from build123d import *

# Parameters (mm, degrees)
CARTRIDGE_BARREL_SKETCH_R         = 16
CARTRIDGE_BARREL_DEPTH            = 17
SIX_MILLIMETRE_FLANGE_SKETCH_R    = 20
SIX_MILLIMETRE_FLANGE_DEPTH       = 6
BEARING_BORE_SKETCH_R             = 14
BEARING_BORE_DEPTH                = 19.6
OUTER_RACE_SHOULDER_EXIT_SKETCH_R = 13
OUTER_RACE_SHOULDER_EXIT_DEPTH    = 3.6
M3_TAPPED_HOLE_PATTERN_SKETCH_R   = 1.5
M3_TAPPED_HOLE_PATTERN_DEPTH      = 6.2


with BuildPart() as part:
    # Cartridge barrel sketch → Cartridge barrel (new body)
    with BuildSketch(Plane(origin=(0, -237.5, 0), x_dir=(1, 0, 0), z_dir=(0, 1, 0))):
        with Locations(Location((-19.009182883, 53.244882879, 0), (0, 0, 270))):
            Circle(CARTRIDGE_BARREL_SKETCH_R)
    extrude(amount=CARTRIDGE_BARREL_DEPTH)

    # Six millimetre flange sketch → Six millimetre flange (add)
    with BuildSketch(Plane(origin=(0, -220.5, 0), x_dir=(1, 0, 0), z_dir=(0, 1, 0))):
        with Locations(Location((-19.009182883, 53.244882879, 0), (0, 0, 270))):
            Circle(SIX_MILLIMETRE_FLANGE_SKETCH_R)
    extrude(amount=SIX_MILLIMETRE_FLANGE_DEPTH)

    # Bearing bore sketch → Bearing bore (cut)
    with BuildSketch(Plane(origin=(0, -237.6, 0), x_dir=(1, 0, 0), z_dir=(0, 1, 0))):
        with Locations(Location((-19.009182883, 53.244882879, 0), (0, 0, 270))):
            Circle(BEARING_BORE_SKETCH_R)
    extrude(amount=BEARING_BORE_DEPTH, mode=Mode.SUBTRACT)

    # Outer race shoulder exit sketch → Outer race shoulder exit (cut)
    with BuildSketch(Plane(origin=(0, -218, 0), x_dir=(1, 0, 0), z_dir=(0, 1, 0))):
        with Locations(Location((-19.009182883, 53.244882879, 0), (0, 0, 270))):
            Circle(OUTER_RACE_SHOULDER_EXIT_SKETCH_R)
    extrude(amount=OUTER_RACE_SHOULDER_EXIT_DEPTH, mode=Mode.SUBTRACT)

    # M3 tapped hole pattern sketch → M3 tapped hole pattern (cut)
    with BuildSketch(Plane(origin=(0, -220.6, 0), x_dir=(1, 0, 0), z_dir=(0, 1, 0))):
        with Locations(Location((-6.493392856, 40.729092852, 0), (0, 0, 270))):
            Circle(M3_TAPPED_HOLE_PATTERN_SKETCH_R)
        with Locations(Location((-31.52497291, 40.729092852, 0), (0, 0, 270))):
            Circle(M3_TAPPED_HOLE_PATTERN_SKETCH_R)
        with Locations(Location((-31.52497291, 65.760672906, 0), (0, 0, 270))):
            Circle(M3_TAPPED_HOLE_PATTERN_SKETCH_R)
        with Locations(Location((-6.493392856, 65.760672906, 0), (0, 0, 270))):
            Circle(M3_TAPPED_HOLE_PATTERN_SKETCH_R)
    extrude(amount=M3_TAPPED_HOLE_PATTERN_DEPTH, mode=Mode.SUBTRACT)


solid = part.part
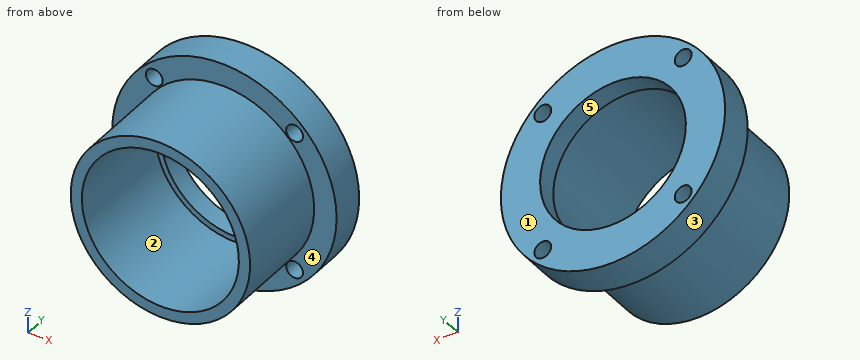
The listing builds one solid part. Answer for the finished solid, in the listing's coordinates (mm). Face numbers are marked on the shaded views. A direction names the side the tool comes from. Round coordinates to 2 decimals unless told otherwise and drop trailing zeros. Write each loop counter-clockwise with the first axis right and the second up, starting at its lowest first coordinate (ties: lowest second). Pieces come first, ordered by that corner, then holes. Notation, with made-up numbers: (15, -30) - (36, -30) arc R18 cw to (36, -20) - close; hole circle Ø10 at (6.5, -8). An arc over 180 degrees is marked (long way). Use a Markdown table: item, result. Add a question column.
1. The part is cut by section A-A (z = -53.5). Write down the section's boundary in (x, y), and give its area (3 significant figures).
2. Flat-ended cylindrical pins translate along their axes: P1, Ø4, axis at y = -227, z = -62.5, coming from the -X side; P2, Ø10, axis at x = -22.5, y = -231, coming from the +Z side; P3, Ø1, axis at x = -16, y = -233.5, coming from the -Z side. Find the tip coordinate at first contact, or state that the pin passes through.
3. The part is cut by section D-D (y = -219.25). Write down the section's boundary in (x, z), and give its area (3 significant figures).
4. The part is cut by section C-C (z = -41). Write down the section's boundary in (x, y).
5. For a pull along X with two mould halves and no side action, classify the marked faces 3, 4 and 5 as +X half, -X half, draft (parallel to the pull), parting line (faces both ways), or undercut.
6. Consider line 1 (Z direction, x = -7, y = -219.75); line 2 (X direction, y = -217.75, z = -67); line 3 (Y direction, x = -7.5, z = -39). Determine where each line is inside the solid, lowest interval first.
7. The part is cut by section B-B (x = -18). Write down the section's boundary in (y, z).
8. A tool of negligible diameter and unlimited length cuts with its end or side. For the marked faces 1 and 2, from which of +Z, -Z, +X, -X, +Y, -Y can it reach the whole face along a straight path? Write none if from no direction.
Reported:
| question | item | result |
|---|---|---|
| 1 | outline | (-39.01, -220.5) - (-35.01, -220.5) - (-35.01, -237.5) - (-33.01, -237.5) - (-33.01, -218) - (-32.01, -218) - (-32.01, -214.5) - (-39.01, -214.5) - close; (-6.01, -218) - (-5.01, -218) - (-5.01, -237.5) - (-3.01, -237.5) - (-3.01, -220.5) - (0.99, -220.5) - (0.99, -214.5) - (-6.01, -214.5) - close |
| 1 | area | 147 mm^2 |
| 2 | P1 | x = -33.27 |
| 2 | P2 | z = -37.24 |
| 2 | P3 | z = -69.05 |
| 3 | outline | circle Ø40 at (-19.01, -53.24); hole circle Ø3 at (-31.52, -65.76); hole circle Ø3 at (-31.52, -40.73); hole circle Ø28 at (-19.01, -53.24); hole circle Ø3 at (-6.49, -65.76); hole circle Ø3 at (-6.49, -40.73) |
| 3 | area | 613 mm^2 |
| 4 | outline | (-34.82, -220.5) - (-33, -220.5) - (-33, -214.5) - (-34.82, -214.5) - close; (-30.05, -220.5) - (-29.31, -220.5) - (-29.31, -237.5) - (-25.8, -237.5) - (-25.8, -218) - (-23.38, -218) - (-23.38, -214.5) - (-30.05, -214.5) - close; (-14.64, -218) - (-12.22, -218) - (-12.22, -237.5) - (-8.71, -237.5) - (-8.71, -220.5) - (-7.97, -220.5) - (-7.97, -214.5) - (-14.64, -214.5) - close; (-5.02, -220.5) - (-3.2, -220.5) - (-3.2, -214.5) - (-5.02, -214.5) - close |
| 5 | face 3 | parting line |
| 5 | face 4 | draft |
| 5 | face 5 | undercut |
| 6 | line 1 | -69.24 to -67.17, -64.35 to -60.44, -46.05 to -42.14, -39.32 to -37.25 |
| 6 | line 2 | -33.53 to -32.37, -30.68 to -7.34, -5.65 to -4.49 |
| 6 | line 3 | -220.5 to -214.5 |
| 7 | outline | (-237.5, -69.21) - (-220.5, -69.21) - (-220.5, -73.22) - (-214.5, -73.22) - (-214.5, -66.21) - (-218, -66.21) - (-218, -67.21) - (-237.5, -67.21) - close; (-237.5, -39.28) - (-218, -39.28) - (-218, -40.28) - (-214.5, -40.28) - (-214.5, -33.27) - (-220.5, -33.27) - (-220.5, -37.28) - (-237.5, -37.28) - close |
| 8 | face 1 | +Z, -Z, +X, -X, +Y |
| 8 | face 2 | -Y |
